Part model, mm, in its own coordinate system. A direction names the side the tool comes from. Round coordinates to 2 decimals unless told otherwise and drop trailing zeros. Loops run counter-clockwise (first coordinate to the right, second up) from the corner with the lowest first, then second, coordinate; pieces in that order, holes last.
(1) Probe probe 1 along X at (y, z) = (16.5, -40.5); probe 2 along X at (y, z) = (15, -36); probe 3 along Y at (x, z) = (0, 32). List the from-to ranges inside material, lowest first.
(2) Flat gauge pins, fed straight in: pin 1 (10 mm diameter, centred on x = 3, y = -4, fed in from +Z) (3 decimals); pin 2 (7.5 mm diameter, centred on x = -5.5, y = 4.5, fed in from +Z) (3 decimals); pin 3 (3.5 mm diameter, centred on x = -15.494, y = 15.494, fed in from +Z); pin 4 (2.5 mm diameter, centred on x = -15.494, y = -15.494, fed in from -Z). Where does each tip first touch, or does it go through?
(3) Cut at D-D on z = 1.5. List the corners of the cut face in (x, y).
(4) Tool access for faces 1 (the face through (-0.33, 2.48, 21.96)), 2 (the face through (0, 21.082, -23)): list every direction of +Z, -Z, +X, -X, +Y, -Y with a clear straight run to the whole face (end or side of a thin tool).
(5) Cut at A-A on z = -15.5. List the corners of the cut face in (x, y).
(6) Cut at B-B on x = 0. List the corners of the cut face in (y, z) (3 decimals), then the cut area to 3 significant figures.
from build123d import *

# Parameters (mm, degrees)
F0_W     = 42.164
F0_H     = 42.164
F1_DEPTH = 47.244
F2_R     = 7.62
F3_R     = 12.7
F4_DEPTH = 3.175
F5_R     = 2.499995
F6_DEPTH = 38.1
F8_DEPTH = 47.245


with BuildPart() as f1:
    # F0 (on Top) → F1 (new body)
    with BuildSketch(Plane.XY):
        Rectangle(F0_W, F0_H)
    extrude(amount=-F1_DEPTH)

    # F2
    f2_edges = [f1.edges().sort_by_distance(p)[0] for p in [
        (21.082, -21.082, -23.622),
        (21.082, 21.082, -23.622),
        (-21.082, 21.082, -23.622),
        (-21.082, -21.082, -23.622),
    ]]
    fillet(f2_edges, radius=F2_R)

    # F3 (on face) → F4 (join)
    with BuildSketch(Plane.XY):
        Circle(F3_R)
    extrude(amount=F4_DEPTH)

    # F5 (on face) → F6 (join)
    with BuildSketch(Plane.XY.offset(3.175)):
        Circle(F5_R)
    extrude(amount=F6_DEPTH)

    # F7 (on face) → F8 (cut, through all)
    with BuildSketch(Plane.XY):
        with BuildLine():
            Line((-15.494, 15.494), (-13.9954, 15.494))
            ThreePointArc((-13.9954, 15.494), (-16.55367, 16.55367), (-15.494, 13.9954))
            Line((-15.494, 13.9954), (-15.494, 15.494))
        make_face()
        with BuildLine():
            ThreePointArc((-15.494, 13.9954), (-14.43433, 14.43433), (-13.9954, 15.494))
            Line((-13.9954, 15.494), (-15.494, 15.494))
            Line((-15.494, 15.494), (-15.494, 13.9954))
        make_face()
        with BuildLine():
            Line((15.494, 15.494), (13.9954, 15.494))
            ThreePointArc((13.9954, 15.494), (14.43433, 14.43433), (15.494, 13.9954))
            Line((15.494, 13.9954), (15.494, 15.494))
        make_face()
        with BuildLine():
            ThreePointArc((16.9926, 15.494), (15.494, 16.9926), (13.9954, 15.494))
            Line((13.9954, 15.494), (15.494, 15.494))
            Line((15.494, 15.494), (15.494, 13.9954))
            ThreePointArc((15.494, 13.9954), (16.55367, 14.43433), (16.9926, 15.494))
        make_face()
        with BuildLine():
            ThreePointArc((16.9926, -15.494), (16.55367, -14.43433), (15.494, -13.9954))
            Line((15.494, -13.9954), (15.494, -15.494))
            Line((15.494, -15.494), (13.9954, -15.494))
            ThreePointArc((13.9954, -15.494), (15.494, -16.9926), (16.9926, -15.494))
        make_face()
        with BuildLine():
            Line((15.494, -15.494), (15.494, -13.9954))
            ThreePointArc((15.494, -13.9954), (14.43433, -14.43433), (13.9954, -15.494))
            Line((13.9954, -15.494), (15.494, -15.494))
        make_face()
        with BuildLine():
            Line((-15.494, -15.494), (-15.494, -13.9954))
            ThreePointArc((-15.494, -13.9954), (-16.55367, -16.55367), (-13.9954, -15.494))
            Line((-13.9954, -15.494), (-15.494, -15.494))
        make_face()
        with BuildLine():
            ThreePointArc((-13.9954, -15.494), (-14.43433, -14.43433), (-15.494, -13.9954))
            Line((-15.494, -13.9954), (-15.494, -15.494))
            Line((-15.494, -15.494), (-13.9954, -15.494))
        make_face()
    extrude(amount=-F8_DEPTH, mode=Mode.SUBTRACT)


solid = f1.part
Final values:
1. probe 1: x = -20.45 to -16.6, -14.38 to 14.38, 16.6 to 20.45
1. probe 2: x = -20.93 to -16.91, -14.08 to 14.08, 16.91 to 20.93
1. probe 3: y = -2.5 to 2.5
2. pin 1: stops at z = 41.275
2. pin 2: stops at z = 3.175
2. pin 3: stops at z = 0
2. pin 4: passes through
3. outline: circle Ø25.4 at (0, 0)
4. face 1: +Z
4. face 2: +Z, -Z, +X, -X, +Y
5. outline: (-21.08, -13.46) arc R7.62 ccw to (-13.46, -21.08) - (13.46, -21.08) arc R7.62 ccw to (21.08, -13.46) - (21.08, 13.46) arc R7.62 ccw to (13.46, 21.08) - (-13.46, 21.08) arc R7.62 ccw to (-21.08, 13.46) - close; hole circle Ø3 at (-15.49, -15.49); hole circle Ø3 at (-15.49, 15.49); hole (14, -15.49) arc R1.5 ccw (long way) to (15.49, -14) arc R1.5 ccw to start; hole (15.49, 14) arc R1.5 ccw to (16.99, 15.49) arc R1.5 ccw (long way) to start
6. outline: (-21.082, -47.244) - (21.082, -47.244) - (21.082, 0) - (12.7, 0) - (12.7, 3.175) - (2.5, 3.175) - (2.5, 41.275) - (-2.5, 41.275) - (-2.5, 3.175) - (-12.7, 3.175) - (-12.7, 0) - (-21.082, 0) - close
6. area: 2,260 mm2
